Geometry: final body of the model. Coordinates: model frame, mm. Face numbers are marked on the shaded views. Round coordinates to 2 decimals unless told otherwise and drop trailing zeros. Loops run counter-clockwise (first coordinate to the right, second up) from the corner with the lowest first, then second, coordinate; pieces in that order, holes last. Notation, with made-up numbers: M -30,-7.75 L 27,-7.75 A25 cw 27,13.25 Z; hole C 69,22 d2. An arc over 180 degrees is marked long. Answer as a JSON object with one key per item and string values.
from build123d import *

# Parameters (mm, degrees)
SKETCH2_R                                      = 15.875
SKETCH2_R_2                                    = 1.7
SKETCH2_R_3                                    = 4
BOSS_EXTRUDE1_DEPTH                            = 2
CSK_FOR_M3_FLAT_HEAD_MACHINE_SCREW2_AT_2_COUNT = 2
CSK_FOR_M3_FLAT_HEAD_MACHINE_SCREW2_AT_2_PITCH = 10.111626971
CSK_FOR_M3_FLAT_HEAD_MACHINE_SCREW2_AT_3_COUNT = 2
CSK_FOR_M3_FLAT_HEAD_MACHINE_SCREW2_AT_3_PITCH = 14.3
CSK_FOR_M3_FLAT_HEAD_MACHINE_SCREW2_AT_4_COUNT = 2
CSK_FOR_M3_FLAT_HEAD_MACHINE_SCREW2_AT_4_PITCH = 10.111626971


with BuildPart() as part:
    # Sketch2 → Boss-Extrude1 (new body)
    with BuildSketch(Plane.XY):
        with Locations((-160.606756626, 98.885631483)):
            Circle(SKETCH2_R)
        with Locations((-165.662570112, 103.941444968)):
            Circle(SKETCH2_R_2, mode=Mode.SUBTRACT)
        with Locations((-155.550943141, 103.941444968)):
            Circle(SKETCH2_R_2, mode=Mode.SUBTRACT)
        with Locations((-155.550943141, 93.829817997)):
            Circle(SKETCH2_R_2, mode=Mode.SUBTRACT)
        with Locations((-165.662570112, 93.829817997)):
            Circle(SKETCH2_R_2, mode=Mode.SUBTRACT)
        with Locations((-160.606756626, 98.885631483)):
            Circle(SKETCH2_R_3, mode=Mode.SUBTRACT)
    extrude(amount=BOSS_EXTRUDE1_DEPTH)

    # Sketch4 → CSK for M3 Flat Head Machine Screw2 (revolve, cut)
    with BuildSketch(Plane(origin=(-165.662570112, 103.941444968, 2), x_dir=(0, -1, 0), z_dir=(1, 0, 0))):
        Polygon((0, 0), (0, 2), (1.7, 2), (1.7, 1.45), (3.15, 0), align=None)
    csk_for_m3_flat_head_machine_screw2 = revolve(axis=Axis((-165.662570112, 103.941444968, 8.35), (0, 0, -1)), mode=Mode.SUBTRACT)

    # CSK for M3 Flat Head Machine Screw2 at 2: CSK for M3 Flat Head Machine Screw2 ×2
    with Locations(*[(i * CSK_FOR_M3_FLAT_HEAD_MACHINE_SCREW2_AT_2_PITCH, 0, 0) for i in range(1, CSK_FOR_M3_FLAT_HEAD_MACHINE_SCREW2_AT_2_COUNT)]):
        add(csk_for_m3_flat_head_machine_screw2, mode=Mode.SUBTRACT)

    # CSK for M3 Flat Head Machine Screw2 at 3: CSK for M3 Flat Head Machine Screw2 ×2
    with Locations(*[Vector(0.707106781, -0.707106781, 0) * (i * CSK_FOR_M3_FLAT_HEAD_MACHINE_SCREW2_AT_3_PITCH) for i in range(1, CSK_FOR_M3_FLAT_HEAD_MACHINE_SCREW2_AT_3_COUNT)]):
        add(csk_for_m3_flat_head_machine_screw2, mode=Mode.SUBTRACT)

    # CSK for M3 Flat Head Machine Screw2 at 4: CSK for M3 Flat Head Machine Screw2 ×2
    with Locations(*[(0, -i * CSK_FOR_M3_FLAT_HEAD_MACHINE_SCREW2_AT_4_PITCH, 0) for i in range(1, CSK_FOR_M3_FLAT_HEAD_MACHINE_SCREW2_AT_4_COUNT)]):
        add(csk_for_m3_flat_head_machine_screw2, mode=Mode.SUBTRACT)


solid = part.part
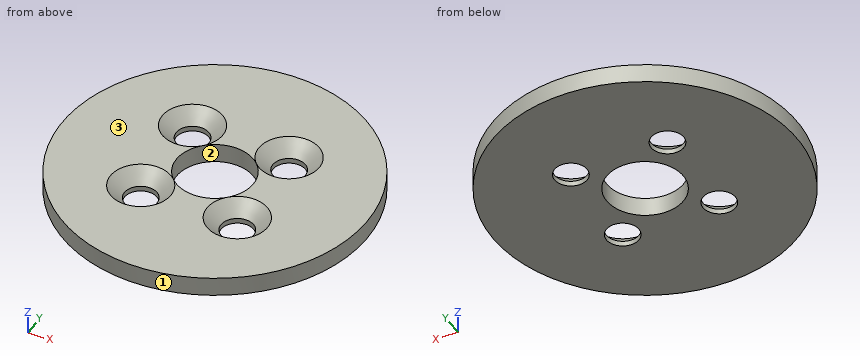
1) Pull-direction query (Y, two-part tool) for the marked faces 1, 2 and 3; classes: +Y half, -Y half, draft (parallel to the pull), parting line (faces both ways), or undercut.
Results:
{"face 1": "parting line", "face 2": "undercut", "face 3": "draft"}
2) Pin query (flat end, axial travel): P1, Ø7, axis at x = -160.61, y = 98.89, coming from the +Z side; P2, Ø5.5, axis at x = -165.66, y = 103.94, coming from the +Z side; P3, Ø10, axis at x = -161, y = 97, coming from the -Z side; P4, Ø1, axis at y = 109, z = 1, coming from the +X side. Return the tip coordinate at first contact, or that it passes through.
Results:
{"P1": "through", "P2": "z = 1.6", "P3": "z = 0", "P4": "x = -147.97"}
3) Section query B-B (y = 98). Return the cut outline in (x, z), and give its area (3 significant figures).
Results:
{"outline": "M -176.46,0 L -164.51,0 L -164.51,2 L -176.46,2 Z; M -156.71,0 L -144.76,0 L -144.76,2 L -156.71,2 Z", "area": "47.8 mm2"}
4) Ray query, line 1 (Y direction, x = -160.5, z = 1.55); line 2 (X direction, y = 105.5, z = 1.55); line 3 (X direction, y = 103.5, z = 0.25). Return the intervals inside material, ascending.
Results:
{"line 1": "83.01 to 94.89, 102.88 to 114.76", "line 2": "-175.04 to -167.87, -163.46 to -157.76, -153.35 to -146.18", "line 3": "-175.8 to -167.3, -164.02 to -157.19, -153.91 to -145.42"}
5) Section query C-C (z = 0.9). Return the cut outline in (x, y) (3 decimals).
Results:
{"outline": "C -160.607,98.886 d31.75; hole C -165.663,93.83 d4.1; hole C -165.663,103.941 d4.1; hole C -160.607,98.886 d8; hole C -155.551,93.83 d4.1; hole C -155.551,103.941 d4.1"}
6) Section query D-D (y = 110). Return the cut outline in (x, z).
Results:
{"outline": "M -171.94,0 L -149.27,0 L -149.27,2 L -171.94,2 Z"}
7) Section query A-A (x = -162). Return the cut outline in (y, z).
Results:
{"outline": "M 83.07,0 L 95.14,0 L 95.14,2 L 83.07,2 Z; M 102.64,0 L 114.7,0 L 114.7,2 L 102.64,2 Z"}
